```python
from build123d import *

# Parameters (mm, degrees)
ESQUISSE1_W             = 40
ESQUISSE1_H             = 57
BOSS_EXTRU_1_DEPTH      = 13.5
ESQUISSE5_W             = 28
ESQUISSE5_H             = 23
ENL_V_MAT_EXTRU_1_DEPTH = 55
ENL_V_MAT_EXTRU_2_REACH = 46.06
ESQUISSE6_R             = 4
ESQUISSE6_3_R           = 7.2
ESQUISSE6_3_R_2         = 5.2
BOSS_EXTRU_2_DEPTH      = 15
ESQUISSE7_W             = 4
ESQUISSE7_H             = 9
ENL_V_MAT_EXTRU_3_DEPTH = 20


with BuildPart() as part:
    # Esquisse1 → Boss.-Extru.1 (new, symmetric)
    with BuildSketch(Plane(origin=(0, 0, 0), x_dir=(1, 0, 0), z_dir=(0, 1, 0))):
        Rectangle(ESQUISSE1_W, ESQUISSE1_H)
    extrude(amount=BOSS_EXTRU_1_DEPTH, both=True)

    # Esquisse5 → Enl_v. mat.-Extru.1 (cut)
    with BuildSketch(Plane.XY.offset(28.5)):
        Rectangle(ESQUISSE5_W, ESQUISSE5_H)
    extrude(amount=-ENL_V_MAT_EXTRU_1_DEPTH, mode=Mode.SUBTRACT)

    # Esquisse6 → Enl_v. mat.-Extru.2 (cut, up to next)
    with BuildSketch(Plane(origin=(0, 13.5, 0), x_dir=(1, 0, 0), z_dir=(0, 1, 0)), mode=Mode.PRIVATE) as enl_v_mat_extru_2_sk1:
        with Locations(Location((0, 0, 0), (0, 0, 270))):
            Circle(ESQUISSE6_R)
    enl_v_mat_extru_2_tool1 = extrude(enl_v_mat_extru_2_sk1.sketch, amount=-ENL_V_MAT_EXTRU_2_REACH, mode=Mode.PRIVATE) & part.part
    add(enl_v_mat_extru_2_tool1.solids().sort_by_distance((0, 13.5, 0))[0], mode=Mode.SUBTRACT)

    # Esquisse6_3 → Boss.-Extru.2 (add)
    with BuildSketch(Plane(origin=(0, 13.5, 0), x_dir=(1, 0, 0), z_dir=(0, 1, 0))):
        with Locations(Location((0, 0, 0), (0, 0, 90))):
            Circle(ESQUISSE6_3_R)
        with Locations(Location((0, 0, 0), (0, 0, 270))):
            Circle(ESQUISSE6_3_R_2, mode=Mode.SUBTRACT)
    extrude(amount=BOSS_EXTRU_2_DEPTH)

    # Esquisse7 → Enl_v. mat.-Extru.3 (cut)
    with BuildSketch(Plane(origin=(0, 13.5, 0), x_dir=(1, 0, 0), z_dir=(0, 1, 0))):
        with Locations((-16, 0)):
            Rectangle(ESQUISSE7_W, ESQUISSE7_H)
    extrude(amount=-ENL_V_MAT_EXTRU_3_DEPTH, mode=Mode.SUBTRACT)


solid = part.part
```
Input: part model. Units: mm. Frame: model coordinates. A direction names the side the tool comes from. Give positions to 0.01 mm unless a question says otherwise; leave off trailing zeros. Order: outer loops, then holes, each group sorted by start corner. A loop starts at its lowest first (then second) coordinate and runs counter-clockwise, first axis right, second up. Notation, with made-up numbers: (20.5, -4.5) - (41.5, -4.5) arc R12 ccw to (41.5, 11.5) - close; hole circle Ø7 at (-28.5, 79). An arc over 180 degrees is marked (long way). Put each result on its own line as item: value.
Item 1: Section query C-C, the plane z = -15. Return loops of the section in (x, y), then the cut area to 3 significant figures.
Found:
outline: (-20, -13.5) - (20, -13.5) - (20, 13.5) - (-20, 13.5) - close; hole (-14, -11.5) - (14, -11.5) - (14, 11.5) - (-14, 11.5) - close
area: 436 mm^2
Item 2: Access query for faces 1 (the flat face through (0, -11.5, 1)), 2 (the flat face through (3, 13.5, 3)), 3 (the flat face through (20, 0, 0)). Directions: +Z, -Z, +X, -X, +Y, -Y. A direction counts if a zero-diameter tool reaches every point of the face in a straight line with its end or side. Return the directions, or none.
Found:
face 1: +Z
face 2: +Y
face 3: +Z, -Z, +X, +Y, -Y
Item 3: Section query B-B, the plane x = 0. Return loops of the section in (y, z), then the cut area to 3 significant figures.
Found:
outline: (-13.5, -28.5) - (13.5, -28.5) - (13.5, -7.2) - (28.5, -7.2) - (28.5, -5.2) - (13.5, -5.2) - (13.5, -4) - (11.5, -4) - (11.5, -26.5) - (-11.5, -26.5) - (-11.5, 28.5) - (-13.5, 28.5) - close; (11.5, 4) - (13.5, 4) - (13.5, 5.2) - (28.5, 5.2) - (28.5, 7.2) - (13.5, 7.2) - (13.5, 28.5) - (11.5, 28.5) - close
area: 318 mm^2
Item 4: Draft query along Z for faces 4 (the cylindrical face through (1.56, 20.9, 4.96)), 5 (the cylindrical face through (2.76, 20.9, -6.65)), 6 (the flat face through (0, 11.5, 7)). Return one class per face: +Z half, -Z half, draft (parallel to the pull), parting line (faces both ways), or undercut.
Found:
face 4: undercut
face 5: parting line
face 6: draft
Item 5: Contact query for flat-ended pins moving along their axis: pin 1 (3 mm diameter, centred on x = -1.5, z = 2.5, fed in from +Y); pin 2 (5 mm diameter, centred on x = 10.5, y = 5.5, fed in from +Z); pin 3 (6 mm diameter, centred on x = 0, z = 0, fed in from +Y). Output: stop coordinate, or through.
Found:
pin 1: stops at y = 13.5
pin 2: stops at z = -26.5
pin 3: stops at y = -11.5
Item 6: Section query A-A, the plane z = 0. Return loops of the section in (x, y).
Found:
outline: (-20, -13.5) - (20, -13.5) - (20, 13.5) - (7.2, 13.5) - (7.2, 28.5) - (5.2, 28.5) - (5.2, 13.5) - (4, 13.5) - (4, 11.5) - (14, 11.5) - (14, -11.5) - (-14, -11.5) - (-14, -6.5) - (-18, -6.5) - (-18, 13.5) - (-20, 13.5) - close; (-14, 11.5) - (-4, 11.5) - (-4, 13.5) - (-5.2, 13.5) - (-5.2, 28.5) - (-7.2, 28.5) - (-7.2, 13.5) - (-14, 13.5) - close
Item 7: Section query D-D, the plane y = 8.5. Return loops of the section in (x, z).
Found:
outline: (-20, -28.5) - (20, -28.5) - (20, 28.5) - (14, 28.5) - (14, -26.5) - (-14, -26.5) - (-14, -4.5) - (-18, -4.5) - (-18, 4.5) - (-14, 4.5) - (-14, 28.5) - (-20, 28.5) - close
Item 8: Ray query, L1, parallel to X at y = 12.2, z = 0; L2, parallel to Y at x = 12, z = 14; L3, parallel to X at y = 17.75, z = 0. Return the intervals inside material, ascending. Write a range as from..to.
Found:
L1: x = -20..-18, -14..-4, 4..20
L2: y = -13.5..-11.5, 11.5..13.5
L3: x = -7.2..-5.2, 5.2..7.2
